Could you check a few things on this model? Use its own coordinates, in mm. Face numbers are marked on the shaded views. A direction names the side the tool comes from. Round coordinates to 2 decimals unless told otherwise and drop trailing zeros. Order: outer loops, then holes, each group sorted by start corner. A loop starts at its lowest first (then second) coordinate and runs counter-clockwise, first axis right, second up. Notation, with made-up numbers: (-14.5, -12) - (0.5, -12) arc R23 cw to (0.5, 0) - close; hole circle Ø6 at (88, 77). An arc over 180 degrees is marked (long way). Use one line per item in the form item = value.
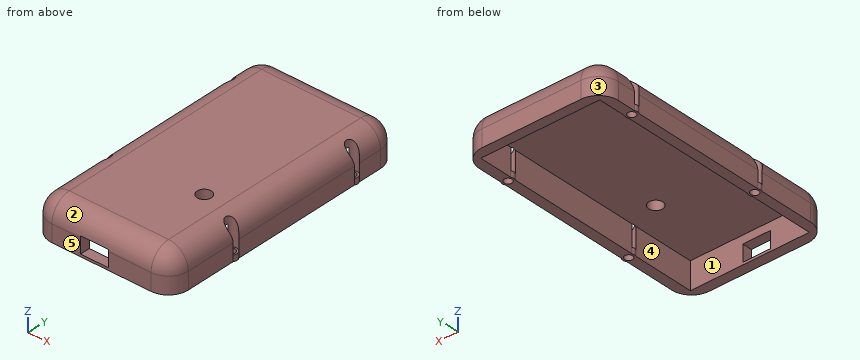
from build123d import *

# Parameters (mm, degrees)
SKETCH1_W           = 70
SKETCH1_H           = 130
BOSS_EXTRUDE1_DEPTH = 18.631112222
SHELL1_T            = -5
FILLET1_R           = 10
FILLET2_R           = 10
FILLET4_R           = 10
FILLET6_R           = 10
SKETCH2_R           = 3.55
CUT_EXTRUDE1_DEPTH  = 26
SKETCH3_W           = 14.110384164
SKETCH3_H           = 8.306919709
CUT_EXTRUDE4_DEPTH  = 30
SKETCH4_R           = 2.85
CUT_EXTRUDE5_DEPTH  = 24
SKETCH5_R           = 2.85
SKETCH5_R_2         = 2
BOSS_EXTRUDE2_DEPTH = 3


with BuildPart() as part:
    # Sketch1 → Boss-Extrude1 (new body)
    with BuildSketch(Plane.XY):
        with Locations((8.736165571, -22.960828507)):
            Rectangle(SKETCH1_W, SKETCH1_H)
    extrude(amount=BOSS_EXTRUDE1_DEPTH)

    # Shell1
    shell1_openings = [part.faces().sort_by_distance(p)[0] for p in [
        (8.736165571, -22.960828507, 0),
    ]]
    offset(amount=SHELL1_T, openings=shell1_openings, kind=Kind.INTERSECTION)

    # Fillet1
    fillet1_edges = [part.edges().sort_by_distance(p)[0] for p in [
        (-26.263834429, -22.960828507, 18.631112222),
    ]]
    fillet(fillet1_edges, radius=FILLET1_R)

    # Fillet2
    fillet2_edges = [part.edges().sort_by_distance(p)[0] for p in [
        (43.736165571, -22.960828507, 18.631112222),
    ]]
    fillet(fillet2_edges, radius=FILLET2_R)

    # Fillet4
    fillet4_edges = [part.edges().sort_by_distance(p)[0] for p in [
        (-26.263834429, 42.039171493, 4.315556111),
        (-23.334902241, 42.039171493, 15.702180034),
        (8.736165571, 42.039171493, 18.631112222),
        (43.736165571, 42.039171493, 4.315556111),
        (40.807233383, 42.039171493, 15.702180034),
    ]]
    fillet(fillet4_edges, radius=FILLET4_R)

    # Fillet6
    fillet6_edges = [part.edges().sort_by_distance(p)[0] for p in [
        (8.736165571, -87.960828507, 18.631112222),
        (-26.263834429, -87.960828507, 4.315556111),
        (-23.334902241, -87.960828507, 15.702180034),
        (43.736165571, -87.960828507, 4.315556111),
        (40.807233383, -87.960828507, 15.702180034),
    ]]
    fillet(fillet6_edges, radius=FILLET6_R)

    # Sketch2 → Cut-Extrude1 (cut)
    with BuildSketch(Plane.XY.offset(7.783233926)):
        with Locations((23.655578881, -46.034025118)):
            Circle(SKETCH2_R)
    extrude(amount=CUT_EXTRUDE1_DEPTH, mode=Mode.SUBTRACT)

    # Sketch3 → Cut-Extrude4 (cut)
    with BuildSketch(Plane(origin=(1.2837e-05, -73.41928233, 3.209e-06), x_dir=(-1, -1.75e-07, 0), z_dir=(1.75e-07, -1, 4.4e-08))):
        with Locations((-5.237013871, -5.398091498)):
            Rectangle(SKETCH3_W, SKETCH3_H)
    extrude(amount=CUT_EXTRUDE4_DEPTH, mode=Mode.SUBTRACT)

    # Sketch4 → Cut-Extrude5 (cut)
    with BuildSketch(Plane.XY):
        with Locations((41.386116272, -50.678340094)):
            Circle(SKETCH4_R)
        with Locations((41.259820466, 18.511183857)):
            Circle(SKETCH4_R)
        with Locations((-23.693524603, -49.042382464)):
            Circle(SKETCH4_R)
        with Locations((-23.751261028, 21.516382028)):
            Circle(SKETCH4_R)
    extrude(amount=CUT_EXTRUDE5_DEPTH, mode=Mode.SUBTRACT)

    # Sketch5 → Boss-Extrude2 (add)
    with BuildSketch(Plane.XY):
        with Locations((-23.751261028, 21.516382028)):
            Circle(SKETCH5_R)
        with Locations((-23.751261028, 21.516382028)):
            Circle(SKETCH5_R_2, mode=Mode.SUBTRACT)
        with Locations((41.259820466, 18.511183857)):
            Circle(SKETCH5_R)
        with Locations((41.259820466, 18.511183857)):
            Circle(SKETCH5_R_2, mode=Mode.SUBTRACT)
        with Locations((41.386116272, -50.678340094)):
            Circle(SKETCH5_R)
        with Locations((41.386116272, -50.678340094)):
            Circle(SKETCH5_R_2, mode=Mode.SUBTRACT)
        with Locations((-23.693524603, -49.042382464)):
            Circle(SKETCH5_R)
        with Locations((-23.693524603, -49.042382464)):
            Circle(SKETCH5_R_2, mode=Mode.SUBTRACT)
    extrude(amount=BOSS_EXTRUDE2_DEPTH)


solid = part.part
Item 1: Imagine slicing it at A-A on z = 7.25. State how many separate pieces and enclosed holes the cut face has, plus the area to 3 significant figures.
Found:
separate_pieces = 5
enclosed_holes = 0
area = 1,650 mm2
Item 2: I need wall thicknesses on L1, parallel to Y at x = 14.5, z = 3.25; L2, parallel to Y at x = 9, z = 5; L3, parallel to X at y = -44, z = 5.5. Which ranges of each line are inside material? Lowest first, please.
Found:
L1 = -87.96 to -82.96, 37.04 to 42.04
L2 = 37.04 to 42.04
L3 = -26.26 to -21.26, 38.74 to 43.74
Item 3: Imagine slicing it at C-C on y = -30. Please give me the cut outline in (x, z), plus the area to 3 significant figures.
Found:
outline = (-26.26, 0) - (-21.26, 0) - (-21.26, 13.63) - (38.74, 13.63) - (38.74, 0) - (43.74, 0) - (43.74, 8.63) arc R10 ccw to (33.74, 18.63) - (-16.26, 18.63) arc R10 ccw to (-26.26, 8.63) - close
area = 443 mm2
Item 4: Will these pins go through, and if not, where does the flat tip stop? P1, Ø1, axis at y = -39, z = 5, coming from the +X side; P2, Ø10, axis at x = 25.5, y = -28.5, coming from the -Z side; P3, Ø1.5, axis at x = 6.5, y = -85.5, coming from the +Z side; P4, Ø3.5, axis at x = -23.75, y = 21.52, coming from the -Z side (3 decimals).
Found:
P1 = 43.74
P2 = 13.63
P3 = 15.97
P4 = through
Item 5: For the marked faces 1 and 2, which set-ups out of +Z, -Z, +X, -X, +Y, -Y let a thin tool reach every point of the face, with its end or its side?
Found:
face_1 = -Z
face_2 = +Z, +X, -X, -Y
Item 6: Imagine slicing it at D-D on x = -8.5. Please give me the cut outline in (y, z).
Found:
outline = (-87.96, 0) - (-82.96, 0) - (-82.96, 13.63) - (37.04, 13.63) - (37.04, 0) - (42.04, 0) - (42.04, 8.63) arc R10 ccw to (32.04, 18.63) - (-77.96, 18.63) arc R10 ccw to (-87.96, 8.63) - close
Item 7: If we mould it in two halves opening along X, with no side actions, what happens to the marked faces 3, 4 and 5? For each: released by +X, released by -X, zero draft, split by the parting line, or undercut.
Found:
face_3 = released by -X
face_4 = undercut
face_5 = zero draft
Item 8: Imagine slicing it at B-B on x = 1. Please give me the cut outline in (y, z).
Found:
outline = (-87.96, 0) - (-82.96, 0) - (-82.96, 1.24) - (-87.96, 1.24) - close; (-87.92, 9.55) - (-82.96, 9.55) - (-82.96, 13.63) - (37.04, 13.63) - (37.04, 0) - (42.04, 0) - (42.04, 8.63) arc R10 ccw to (32.04, 18.63) - (-77.96, 18.63) arc R10 ccw to start
